Job drawing, mm, ordinate dimensions from the low corner. One solid piece. Coordinates: 2 decimals unless noted, no trailing zeros. Write each loop counter-clockwise with the first axis right and the second up, starting at its lowest first coordinate (ties: lowest second). Pieces come first, ordered by that corner, then holes. Notation, with made-up numbers: (-17.75, 61) - (2.25, 61) arc R22 cw to (2.25, 68) - close; hole circle Ø5 at (-14, 51.25). An arc over 180 degrees is marked (long way). Use a Markdown table: item, result.
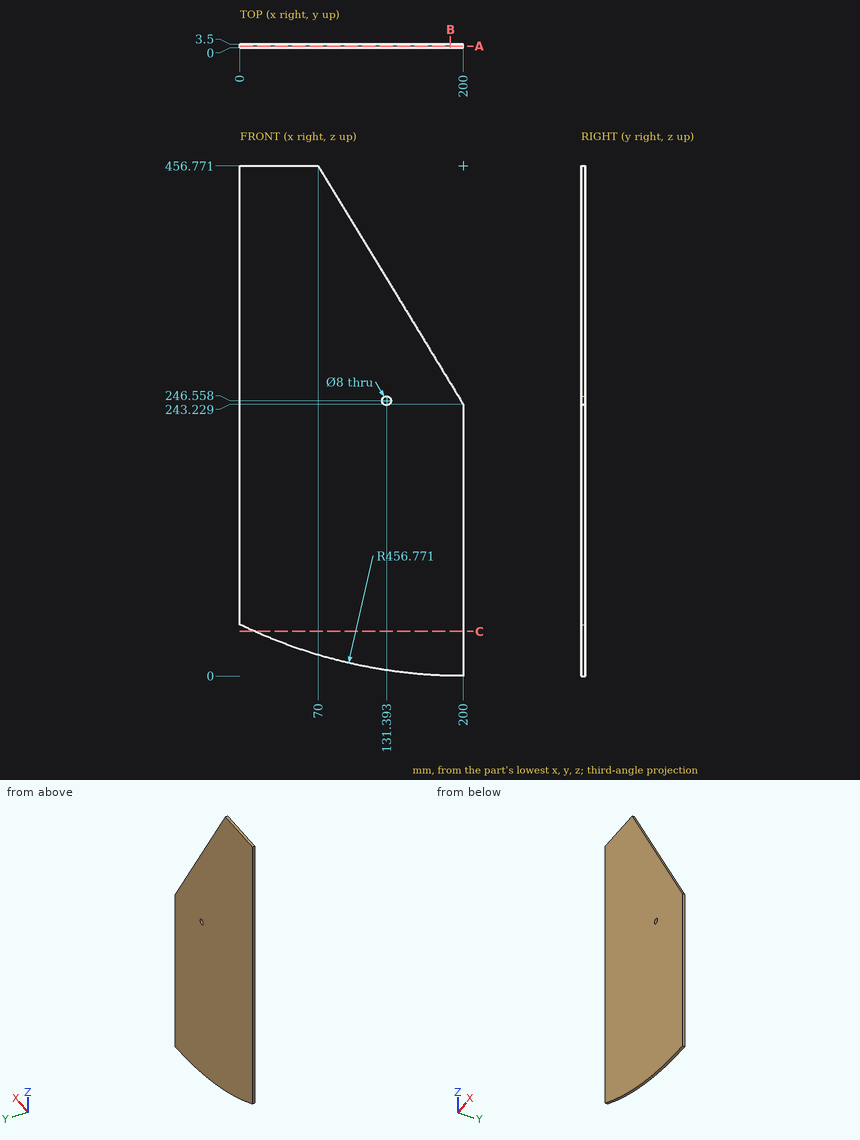
Item 1: Band-saw the part on A-A, the plane y = 1.65. Give the cut face in (x, z).
From the geometry:
| item | result |
|---|---|
| outline | (0, 46.11) arc R456.77 ccw to (200, 0) - (200, 243.23) - (70, 456.77) - (0, 456.77) - close; hole circle Ø8 at (131.39, 246.56) |
Item 2: Band-saw the part on C-C, the plane z = 40. Give the cut face in (x, y), then the cut area to 3 significant figures.
From the geometry:
| item | result |
|---|---|
| outline | (13.07, 0) - (200, 0) - (200, 3.5) - (13.07, 3.5) - close |
| area | 654 mm^2 |
Item 3: Drop a flat-ended pin along its axis: P1, Ø2, axis at x = 171, z = 253, coming from the -Y side. Give the stop position or say it passes through.
From the geometry:
| item | result |
|---|---|
| P1 | y = 0 |
Item 4: Drill centre lines: probe 1 along Z at (x, y) = (130, 1.95) (1 decimal); probe 2 along X at (y, z) = (1.5, 250) (1 decimal); probe 3 along Z at (x, y) = (13, 0.5). Where is each one in solid material? Low to high.
From the geometry:
| item | result |
|---|---|
| probe 1 | 5.4 to 242.8, 250.3 to 358.2 |
| probe 2 | 0 to 129.4, 133.4 to 195.9 |
| probe 3 | 40.03 to 456.77 |
Item 5: Band-saw the part on B-B, the plane x = 188.5. Give the cut face in (y, z) (1 decimal), then the cut area to 3 significant figures.
From the geometry:
| item | result |
|---|---|
| outline | (0, 0.1) - (3.5, 0.1) - (3.5, 262.1) - (0, 262.1) - close |
| area | 917 mm^2 |
